```python
from build123d import *
from build123d.topology import SkipClean

# Parameters (mm, degrees)
BOSS_EXTRUDE1_DEPTH     = 3
BOSS_EXTRUDE2_DEPTH     = 2.5
CHAMFER1_SIZE           = 2
CHAMFER1_SIZE2          = 3.464101615
CHAMFER2_SIZE           = 2
CHAMFER2_SIZE2          = 3.464101615
CUT_EXTRUDE1_START      = -2.5
CUT_EXTRUDE1_DEPTH      = 2.5
CUT_EXTRUDE2_DEPTH      = 42.632739521
CUT_EXTRUDE2_DEPTH_BACK = 42.632739521
SKETCH4_R               = 17.222950649
SKETCH4_R_2             = 13.5
CUT_EXTRUDE3_DEPTH      = 42.409207913
CUT_EXTRUDE3_DEPTH_BACK = 42.409207913
FILLET1_R               = 1.5


with BuildPart() as part:
    # Sketch1 → Boss-Extrude1 (new body)
    with BuildSketch(Plane.XY):
        with BuildLine():
            Line((-33.222718241, -2.222718241), (-31.172108576, -0.172108576))
            ThreePointArc((-31.172108576, -0.172108576), (-34.35, 7.5), (-31.172108576, 15.172108576))
            Line((-31.172108576, 15.172108576), (-33.222718241, 17.222718241))
            ThreePointArc((-33.222718241, 17.222718241), (-37.25, 7.5), (-33.222718241, -2.222718241))
        make_face()
        with BuildLine():
            Line((-31.172108576, -0.172108576), (-29.863961031, 1.136038969))
            ThreePointArc((-29.863961031, 1.136038969), (-32.5, 7.5), (-29.863961031, 13.863961031))
            Line((-29.863961031, 13.863961031), (-31.172108576, 15.172108576))
            ThreePointArc((-31.172108576, 15.172108576), (-34.35, 7.5), (-31.172108576, -0.172108576))
        make_face()
        with BuildLine():
            ThreePointArc((-29.863961031, 13.863961031), (-26.944150891, 15.814915793), (-23.5, 16.5))
            Line((-23.5, 16.5), (-23.5, 18.35))
            ThreePointArc((-23.5, 18.35), (-27.652115241, 17.524092928), (-31.172108576, 15.172108576))
            Line((-31.172108576, 15.172108576), (-29.863961031, 13.863961031))
        make_face()
        with BuildLine():
            Line((-23.5, 18.35), (-23.5, 16.5))
            ThreePointArc((-23.5, 16.5), (-20.055849109, 15.814915793), (-17.136038969, 13.863961031))
            Line((-17.136038969, 13.863961031), (-15.827891424, 15.172108576))
            ThreePointArc((-15.827891424, 15.172108576), (-19.347884759, 17.524092928), (-23.5, 18.35))
        make_face()
        with BuildLine():
            Line((-15.827891424, 15.172108576), (-17.136038969, 13.863961031))
            ThreePointArc((-17.136038969, 13.863961031), (-15.185084207, 10.944150891), (-14.5, 7.5))
            ThreePointArc((-14.5, 7.5), (-15.185084207, 4.055849109), (-17.136038969, 1.136038969))
            Line((-17.136038969, 1.136038969), (-15.827891424, -0.172108576))
            ThreePointArc((-15.827891424, -0.172108576), (-13.475907072, 3.347884759), (-12.65, 7.5))
            ThreePointArc((-12.65, 7.5), (-13.475907072, 11.652115241), (-15.827891424, 15.172108576))
        make_face()
        with BuildLine():
            ThreePointArc((-17.136038969, 1.136038969), (-20.055849109, -0.814915793), (-23.5, -1.5))
            Line((-23.5, -1.5), (-23.5, -3.35))
            ThreePointArc((-23.5, -3.35), (-19.347884759, -2.524092928), (-15.827891424, -0.172108576))
            Line((-15.827891424, -0.172108576), (-17.136038969, 1.136038969))
        make_face()
        with BuildLine():
            Line((-23.5, -3.35), (-23.5, -1.5))
            ThreePointArc((-23.5, -1.5), (-26.944150891, -0.814915793), (-29.863961031, 1.136038969))
            Line((-29.863961031, 1.136038969), (-31.172108576, -0.172108576))
            ThreePointArc((-31.172108576, -0.172108576), (-27.652115241, -2.524092928), (-23.5, -3.35))
        make_face()
        with BuildLine():
            Line((-13.777281759, 17.222718241), (-15.827891424, 15.172108576))
            ThreePointArc((-15.827891424, 15.172108576), (-13.475907072, 11.652115241), (-12.65, 7.5))
            ThreePointArc((-12.65, 7.5), (-13.475907072, 3.347884759), (-15.827891424, -0.172108576))
            Line((-15.827891424, -0.172108576), (-13.777281759, -2.222718241))
            ThreePointArc((-13.777281759, -2.222718241), (-10.796656428, 2.238102805), (-9.75, 7.5))
            ThreePointArc((-9.75, 7.5), (-10.796656428, 12.761897195), (-13.777281759, 17.222718241))
        make_face()
    extrude(amount=BOSS_EXTRUDE1_DEPTH)

    # Sketch2 → Boss-Extrude2 (add)
    with BuildSketch(Plane.XY.offset(3)):
        with BuildLine():
            Line((-37.25, 7.5), (-32.5, 7.5))
            ThreePointArc((-32.5, 7.5), (-31.814915793, 10.944150891), (-29.863961031, 13.863961031))
            Line((-29.863961031, 13.863961031), (-31.172108576, 15.172108576))
            Line((-31.172108576, 15.172108576), (-33.222718241, 17.222718241))
            ThreePointArc((-33.222718241, 17.222718241), (-36.203343572, 12.761897195), (-37.25, 7.5))
        make_face()
        with BuildLine():
            Line((-9.75, 7.5), (-14.5, 7.5))
            ThreePointArc((-14.5, 7.5), (-15.185084207, 4.055849109), (-17.136038969, 1.136038969))
            Line((-17.136038969, 1.136038969), (-15.827891424, -0.172108576))
            Line((-15.827891424, -0.172108576), (-13.777281759, -2.222718241))
            ThreePointArc((-13.777281759, -2.222718241), (-10.796656428, 2.238102805), (-9.75, 7.5))
        make_face()
    extrude(amount=BOSS_EXTRUDE2_DEPTH)

    # Chamfer1
    chamfer1_edges = [part.edges().sort_by_distance(p)[0] for p in [
        (-32.197413409, -1.197413409, 3),
    ]]
    chamfer1_side = [part.faces().sort_by_distance(p)[0] for p in [
        (-32.197413409, -1.197413409, 1.5),
    ]]
    chamfer(chamfer1_edges, length=CHAMFER1_SIZE, length2=CHAMFER1_SIZE2, reference=chamfer1_side[0])

    # Chamfer2
    chamfer2_edges = [part.edges().sort_by_distance(p)[0] for p in [
        (-14.802586591, 16.197413409, 3),
    ]]
    chamfer2_side = [part.faces().sort_by_distance(p)[0] for p in [
        (-14.802586591, 16.197413409, 1.5),
    ]]
    chamfer(chamfer2_edges, length=CHAMFER2_SIZE, length2=CHAMFER2_SIZE2, reference=chamfer2_side[0])

    # Sketch3 → Cut-Extrude1 (cut)
    with BuildSketch(Plane.XY.offset(5.5).offset(CUT_EXTRUDE1_START)):
        with BuildLine():
            Line((-11.038267928, 1.688998901), (-15.343229917, 3.696435644))
            ThreePointArc((-15.343229917, 3.696435644), (-16.127631601, 2.337812073), (-17.136038969, 1.136038969))
            Line((-17.136038969, 1.136038969), (-13.777281759, -2.222718241))
            ThreePointArc((-13.777281759, -2.222718241), (-12.236659391, -0.386676), (-11.038267928, 1.688998901))
        make_face()
        with BuildLine():
            Line((-35.961732072, 13.311001099), (-31.656770083, 11.303564356))
            ThreePointArc((-31.656770083, 11.303564356), (-30.872368399, 12.662187927), (-29.863961031, 13.863961031))
            Line((-29.863961031, 13.863961031), (-33.222718241, 17.222718241))
            ThreePointArc((-33.222718241, 17.222718241), (-34.763340609, 15.386676), (-35.961732072, 13.311001099))
        make_face()
    extrude(amount=CUT_EXTRUDE1_DEPTH, mode=Mode.SUBTRACT)

    # Sketch4 → Cut-Extrude2 (cut, two sides: drawn at the far end of the back side and taken through both)
    with BuildSketch(Plane.XY.offset(3).offset(-CUT_EXTRUDE2_DEPTH_BACK)):
        with Locations((-23.5, 7.5)):
            Circle(SKETCH4_R)
        with Locations((-23.5, 7.5)):
            Circle(SKETCH4_R_2, mode=Mode.SUBTRACT)
    extrude(amount=CUT_EXTRUDE2_DEPTH + CUT_EXTRUDE2_DEPTH_BACK, mode=Mode.SUBTRACT)

    # Sketch5 → Cut-Extrude3 (cut, two sides: drawn at the far end of the back side and taken through both)
    with SkipClean():  # the faces are left unmerged after this step: merging them gives an invalid solid
        with BuildSketch(Plane.XY.offset(3).offset(-CUT_EXTRUDE3_DEPTH_BACK)):
            with BuildLine():
                Line((-33.373274972, 16.706977861), (-31.435187663, 14.899682207))
                ThreePointArc((-31.435187663, 14.899682207), (-31.304836834, 15.037043319), (-31.172108576, 15.172108576))
                Line((-31.172108576, 15.172108576), (-33.045941546, 17.045941546))
                ThreePointArc((-33.045941546, 17.045941546), (-33.211087305, 16.877888001), (-33.373274972, 16.706977861))
            make_face()
            with BuildLine():
                Line((-13.626725028, -1.706977861), (-15.564812337, 0.100317793))
                ThreePointArc((-15.564812337, 0.100317793), (-15.695163166, -0.037043319), (-15.827891424, -0.172108576))
                Line((-15.827891424, -0.172108576), (-13.954058454, -2.045941546))
                ThreePointArc((-13.954058454, -2.045941546), (-13.788912695, -1.877888001), (-13.626725028, -1.706977861))
            make_face()
        extrude(amount=CUT_EXTRUDE3_DEPTH + CUT_EXTRUDE3_DEPTH_BACK, mode=Mode.SUBTRACT)

    # Fillet1
    fillet1_edges = [part.edges().sort_by_distance(p)[0] for p in [
        (-13.304037396, 2.745544555, 5.5),
        (-33.695962604, 12.254455445, 5.5),
        (-10.320003904, 4.578065212, 5.5),
        (-36.679996096, 10.421934788, 5.5),
        (-34.75, 7.5, 5.5),
        (-32.286664064, 9.447956525, 5.5),
        (-12.25, 7.5, 5.5),
        (-14.713335936, 5.552043475, 5.5),
    ]]
    fillet(fillet1_edges, radius=FILLET1_R)


solid = part.part
```
Could you check a few things on this model? Use its own coordinates, in mm. A direction names the side the tool comes from. Round coordinates to 2 decimals unless told otherwise and drop trailing zeros. Loops run counter-clockwise (first coordinate to the right, second up) from the corner with the lowest first, then second, coordinate; pieces in that order, holes last. Notation, with made-up numbers: M 48.5,-17 L 102.5,-17 A12 ccw 102.5,-11 Z; hole C -8.75,38 d2. An arc over 180 degrees is marked long. Write item = value, one per line.
1. I need wall thicknesses on probe 1 along X at (y, z) = (15.5, 2.9); probe 2 along Y at (x, z) = (-23.5, 2.7); probe 3 along Z at (x, y) = (-35, 1). Which ranges of each line are inside material? Lowest first, please.
Results below:
probe_1 = -34.37 to -32.08, -30.83 to -27.62, -19.38 to -16.17
probe_2 = -3.35 to -1.5, 16.5 to 18.35
probe_3 = 0 to 3
2. I want a section at A-A, the plane z = 0.6. Write out the boundary of the cut face in (x, y).
Results below:
outline = M -33.37,16.71 A13.5 ccw -33.05,-2.05 L -31.17,-0.17 A10.85 ccw -15.83,-0.17 A10.85 ccw -15.56,0.1 L -13.63,-1.71 A13.5 ccw -13.95,17.05 L -15.83,15.17 A10.85 ccw -31.17,15.17 A10.85 ccw -31.44,14.9 Z; hole C -23.5,7.5 d18
3. I want a section at B-B, the plane z = 3.7. Write out the boundary of the cut face in (x, y), and give its area (3 significant figures).
Results below:
outline = M -37,7.5 L -32.5,7.5 A9 cw -31.66,11.3 L -35.74,13.21 A13.5 ccw Z; M -15.34,3.7 L -11.26,1.79 A13.5 ccw -10,7.5 L -14.5,7.5 A9 cw Z
area = 44.2 mm²
4. I want a section at D-D, the plane y = 1.5. Write out the boundary of the cut face in (x, z).
Results below:
outline = M -35.59,0 L -30.21,0 L -30.21,3 L -32.54,3 L -32.54,2.24 L -34.4,3 L -35.59,3 Z; M -16.79,0 L -11.41,0 L -11.41,3 L -16.79,3 Z
5. Will these pins go through, and if not, where does the flat tip stop? P1, Ø3.5, axis at x = -19, y = 4.5, coming from the +Z side; P2, Ø3, axis at x = -17.5, y = 0.5, coming from the +Z side; P3, Ø8, axis at x = -16.5, y = 0.5, coming from the +Z side.
Results below:
P1 = through
P2 = 3
P3 = 5.2
6. Thinking about a two-plate mould opening in X: for faces 1 (the face through (-13.834, 14.682, 2.014)), 2 (the face through (-12.2, 7.5, 3.5)), 3 (the face through (-13.275, 2.732, 3.493)), which applies, +X half, -X half, draft (parallel to the pull), parting line (faces both ways), or undercut?
Results below:
face_1 = undercut
face_2 = draft
face_3 = -X half
7. Which directions (+Z, -Z, +X, -X, +Y, -Y) give clear straight access to the entire face, cutting with the end or side of a thin tool? Please do faces 4 (the face through (-33.166, 0.318, 2.014)), 5 (the face through (-14.6, -0.8, 1.5)), 6 (the face through (-32.4, 15.8, 1.5)), 7 (the face through (-28, -1, 3)), 8 (the face through (-21, 17, 3)).
Results below:
face_4 = +Z, -Y
face_5 = +Z, -Z, -Y
face_6 = +Z, -Z, +Y
face_7 = +Z, -X, -Y
face_8 = +Z, +X, +Y
8. I want a section at C-C, the plane x = -21.25. Write out the boundary of the cut face in (y, z), and give its area (3 significant figures).
Results below:
outline = M -3.11,0 L -1.21,0 L -1.21,3 L -3.11,3 Z; M 16.21,0 L 18.11,0 L 18.11,3 L 16.21,3 Z
area = 11.4 mm²
